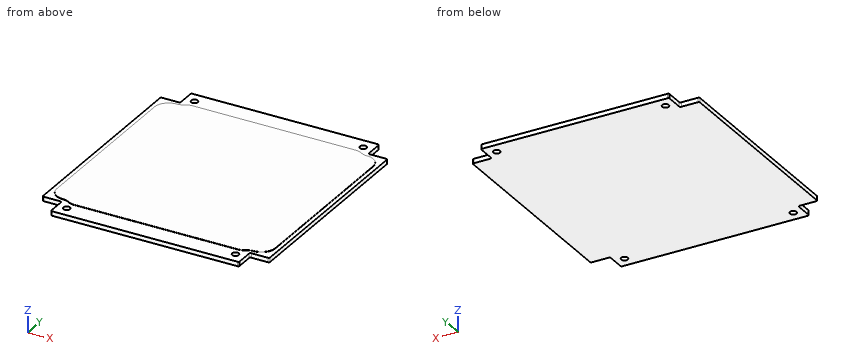
from build123d import *

# Parameters (mm, degrees)
BOSS_EXTRUDE1_DEPTH            = 1.6
BOSS_EXTRUDE2_DEPTH            = 0.1
M2_HOLE1_FIXINGSTRUCTURE_D     = 2.4
M2_HOLE1_FIXINGSTRUCTURE_DEPTH = 200
M2_HOLE1_FIXINGSTRUCTURE_TIP   = 0.721032743


with BuildPart() as part:
    # Sketch1 → Boss-Extrude1 (new body)
    with BuildSketch(Plane.XY):
        with BuildLine():
            Line((-34, 44), (-34, 38))
            ThreePointArc((-34, 38), (-34.146446609, 37.646446609), (-34.5, 37.5))
            Line((-34.5, 37.5), (-40.5, 37.5))
            ThreePointArc((-40.5, 37.5), (-40.853553391, 37.353553391), (-41, 37))
            Line((-41, 37), (-41, -37))
            ThreePointArc((-41, -37), (-40.853553391, -37.353553391), (-40.5, -37.5))
            Line((-40.5, -37.5), (-34.5, -37.5))
            ThreePointArc((-34.5, -37.5), (-34.146446609, -37.646446609), (-34, -38))
            Line((-34, -38), (-34, -44))
            ThreePointArc((-34, -44), (-33.853553391, -44.353553391), (-33.5, -44.5))
            Line((-33.5, -44.5), (33.5, -44.5))
            ThreePointArc((33.5, -44.5), (33.853553391, -44.353553391), (34, -44))
            Line((34, -44), (34, -38))
            ThreePointArc((34, -38), (34.146446609, -37.646446609), (34.5, -37.5))
            Line((34.5, -37.5), (40.5, -37.5))
            ThreePointArc((40.5, -37.5), (40.853553391, -37.353553391), (41, -37))
            Line((41, -37), (41, 37))
            ThreePointArc((41, 37), (40.853553391, 37.353553391), (40.5, 37.5))
            Line((40.5, 37.5), (34.5, 37.5))
            ThreePointArc((34.5, 37.5), (34.146446609, 37.646446609), (34, 38))
            Line((34, 38), (34, 44))
            ThreePointArc((34, 44), (33.853553391, 44.353553391), (33.5, 44.5))
            Line((33.5, 44.5), (-33.5, 44.5))
            ThreePointArc((-33.5, 44.5), (-33.853553391, 44.353553391), (-34, 44))
        make_face()
    extrude(amount=BOSS_EXTRUDE1_DEPTH)

    # Esboço1 → Boss-Extrude2 (add)
    with BuildSketch(Plane.XY.offset(1.6)):
        with BuildLine():
            Line((-29.5, -37.5), (29.5, -37.5))
            ThreePointArc((29.5, -37.5), (30.805038314, -37.308461045), (32, -36.75))
            ThreePointArc((32, -36.75), (33.194961686, -36.191538955), (34.5, -36))
            ThreePointArc((34.5, -36), (38.035533906, -34.535533906), (39.5, -31))
            Line((39.5, -31), (39.5, 31))
            ThreePointArc((39.5, 31), (38.035533906, 34.535533906), (34.5, 36))
            ThreePointArc((34.5, 36), (33.194961686, 36.191538955), (32, 36.75))
            ThreePointArc((32, 36.75), (30.805038314, 37.308461045), (29.5, 37.5))
            Line((29.5, 37.5), (-29.5, 37.5))
            ThreePointArc((-29.5, 37.5), (-30.805038314, 37.308461045), (-32, 36.75))
            ThreePointArc((-32, 36.75), (-33.194961686, 36.191538955), (-34.5, 36))
            ThreePointArc((-34.5, 36), (-38.035533906, 34.535533906), (-39.5, 31))
            Line((-39.5, 31), (-39.5, -31))
            ThreePointArc((-39.5, -31), (-38.035533906, -34.535533906), (-34.5, -36))
            ThreePointArc((-34.5, -36), (-33.194961686, -36.191538955), (-32, -36.75))
            ThreePointArc((-32, -36.75), (-30.805038314, -37.308461045), (-29.5, -37.5))
        make_face()
    extrude(amount=BOSS_EXTRUDE2_DEPTH)

    # M2 Hole1-FixingStructure
    with Locations(Plane(origin=(0, 0, 0), x_dir=(-1, 0, 0), z_dir=(0, 0, -1))):
        with Locations((-30.5, 40.5), (30.5, 40.5), (-30.5, -40.5), (30.5, -40.5)):
            Hole(M2_HOLE1_FIXINGSTRUCTURE_D / 2, depth=M2_HOLE1_FIXINGSTRUCTURE_DEPTH)
            with Locations((0, 0, -(M2_HOLE1_FIXINGSTRUCTURE_DEPTH + M2_HOLE1_FIXINGSTRUCTURE_TIP / 2))):  # 118° drill point
                Cone(0, M2_HOLE1_FIXINGSTRUCTURE_D / 2, M2_HOLE1_FIXINGSTRUCTURE_TIP, mode=Mode.SUBTRACT)


solid = part.part
Check sheet for the modelled part. Datum: model origin and axes. Units: mm. Give positions to 0.01 mm unless a question says otherwise; leave off trailing zeros. Loops run counter-clockwise (first coordinate to the right, second up) from the corner with the lowest first, then second, coordinate; pieces in that order, holes last. Notation, with made-up numbers: M 22.5,68 L 36.5,68 A7 ccw 36.5,79 Z; hole C -31,-3 d11. An arc over 180 degrees is marked long. Use a Markdown table: item, result. Add a question column.
Q1. Sectioned sample at B-B, the plane x = 30.5. Record the cut outline in (y, z).
Q2. Go/stop test with flat-tipped pins: pin 1 (0.8 mm diameter, centred on y = -41.5, z = 1, fed in from +X); pin 2 (2 mm diameter, centred on x = 30.5, y = 40.5, fed in from +Z); pin 3 (10 mm diameter, centred on x = -32, y = 15, fed in from -Z); pin 4 (0.5 mm diameter, centred on x = -38.5, z = 0.5, fed in from -Y). Record where each tip stops, or that it passes through.
Q3. Sectioned sample at C-C, the plane z = 0.7. Record the cut outline in (x, y), then the cut area to 3 significant figures.
Q4. Scan lines: line 1 along Y through (x, z) = (-30.5, 0.45); line 2 along Y through (x, z) = (31, 0.15); line 3 along Y through (x, z) = (37.5, 1.55). Record each from-to range of solid material in increasing order. Write a range as [from, to].
Q5. Sectioned sample at A-A, the plane y = 40.5. Record the cut outline in (x, z).
Verdict:
| question | item | result |
|---|---|---|
| 1 | outline | M -44.5,0 L -41.7,0 L -41.7,1.6 L -44.5,1.6 Z; M -39.3,0 L 39.3,0 L 39.3,1.6 L 37.39,1.6 L 37.39,1.7 L -37.39,1.7 L -37.39,1.6 L -39.3,1.6 Z; M 41.7,0 L 44.5,0 L 44.5,1.6 L 41.7,1.6 Z |
| 2 | pin 1 | x = 34 |
| 2 | pin 2 | through |
| 2 | pin 3 | z = 0 |
| 2 | pin 4 | y = -37.5 |
| 3 | outline | M -41,-37 A0.5 ccw -40.5,-37.5 L -34.5,-37.5 A0.5 cw -34,-38 L -34,-44 A0.5 ccw -33.5,-44.5 L 33.5,-44.5 A0.5 ccw 34,-44 L 34,-38 A0.5 cw 34.5,-37.5 L 40.5,-37.5 A0.5 ccw 41,-37 L 41,37 A0.5 ccw 40.5,37.5 L 34.5,37.5 A0.5 cw 34,38 L 34,44 A0.5 ccw 33.5,44.5 L -33.5,44.5 A0.5 ccw -34,44 L -34,38 A0.5 cw -34.5,37.5 L -40.5,37.5 A0.5 ccw -41,37 Z; hole C -30.5,-40.5 d2.4; hole C -30.5,40.5 d2.4; hole C 30.5,-40.5 d2.4; hole C 30.5,40.5 d2.4 |
| 3 | area | 7,080 mm^2 |
| 4 | line 1 | [-44.5, -41.7], [-39.3, 39.3], [41.7, 44.5] |
| 4 | line 2 | [-44.5, -41.59], [-39.41, 39.41], [41.59, 44.5] |
| 4 | line 3 | [-37.5, 37.5] |
| 5 | outline | M -34,0 L -31.7,0 L -31.7,1.6 L -34,1.6 Z; M -29.3,0 L 29.3,0 L 29.3,1.6 L -29.3,1.6 Z; M 31.7,0 L 34,0 L 34,1.6 L 31.7,1.6 Z |
